The listing builds one solid part. Answer for the finished solid, in the listing's coordinates (mm). Coordinates: 2 decimals unless noted, no trailing zeros. Order: outer loops, then holes, each group sorted by start corner. A loop starts at its lowest first (then second) coordinate and runs counter-clockwise, first axis right, second up. Notation, with made-up numbers: (89, -36) -> (102, -36) arc R21 ccw to (102, -10) -> close; hole circle Ø4 at (63, 1). An arc over 180 degrees is marked (long way). Answer in a Markdown table with one row per item.
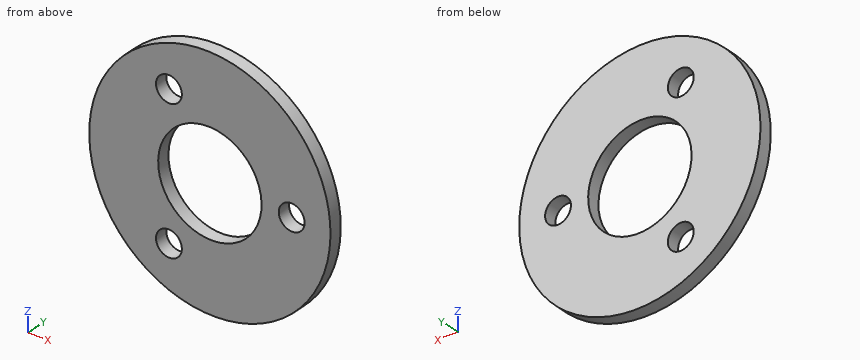
```python
from build123d import *

# Parameters (mm, degrees)
SKETCH_1_R          = 14
SKETCH_1_R_2        = 6
EXTRUDE_1_DEPTH     = 1.5
CUT_EXTRUDE_2_REACH = 21.856
SKETCH_2_R          = 1.5


with BuildPart() as part:
    # 草图1 → 凸台-拉伸1 (new body)
    with BuildSketch(Plane(origin=(0, 0, 0), x_dir=(1, 0, 0), z_dir=(0, 1, 0))):
        with Locations(Location((0, 0, 0), (0, 0, 270))):
            Circle(SKETCH_1_R)
        with Locations(Location((0, 0, 0), (0, 0, 270))):
            Circle(SKETCH_1_R_2, mode=Mode.SUBTRACT)
    extrude(amount=EXTRUDE_1_DEPTH)

    # 草图2 → 切除-拉伸2 (cut, up to next)
    with BuildSketch(Plane(origin=(0, 0, 0), x_dir=(1, 0, 0), z_dir=(0, 1, 0)), mode=Mode.PRIVATE) as cut_extrude_2_sk1:
        with Locations(Location((9.5, 0, 0), (0, 0, 270))):
            Circle(SKETCH_2_R)
    cut_extrude_2_tool1 = extrude(cut_extrude_2_sk1.sketch, amount=CUT_EXTRUDE_2_REACH, mode=Mode.PRIVATE) & part.part
    # 草图2 → 切除-拉伸2 (cut, up to next)
    with BuildSketch(Plane(origin=(0, 0, 0), x_dir=(1, 0, 0), z_dir=(0, 1, 0)), mode=Mode.PRIVATE) as cut_extrude_2_sk2:
        with Locations(Location((-4.75, -8.227241336, 0), (0, 0, 270))):
            Circle(SKETCH_2_R)
    cut_extrude_2_tool2 = extrude(cut_extrude_2_sk2.sketch, amount=CUT_EXTRUDE_2_REACH, mode=Mode.PRIVATE) & part.part
    # 草图2 → 切除-拉伸2 (cut, up to next)
    with BuildSketch(Plane(origin=(0, 0, 0), x_dir=(1, 0, 0), z_dir=(0, 1, 0)), mode=Mode.PRIVATE) as cut_extrude_2_sk3:
        with Locations(Location((-4.75, 8.227241336, 0), (0, 0, 270))):
            Circle(SKETCH_2_R)
    cut_extrude_2_tool3 = extrude(cut_extrude_2_sk3.sketch, amount=CUT_EXTRUDE_2_REACH, mode=Mode.PRIVATE) & part.part
    add(cut_extrude_2_tool1.solids().sort_by_distance((9.5, 0, 0))[0], mode=Mode.SUBTRACT)
    add(cut_extrude_2_tool2.solids().sort_by_distance((-4.75, 0, 8.227241))[0], mode=Mode.SUBTRACT)
    add(cut_extrude_2_tool3.solids().sort_by_distance((-4.75, 0, -8.227241))[0], mode=Mode.SUBTRACT)


solid = part.part
```
(1) Find the intervals of material crossed by line 1 along X through (y, z) = (1.3, 0); line 2 along Z through (x, y) = (-4.75, 0.45); line 3 along Z through (x, y) = (9.5, 0.75), in increasing order. Write a range as from..to.
Check values:
| item | result |
|---|---|
| line 1 | -14..-6, 6..8, 11..14 |
| line 2 | -13.17..-9.73, -6.73..-3.67, 3.67..6.73, 9.73..13.17 |
| line 3 | -10.28..-1.5, 1.5..10.28 |
(2) A cutting plane is placed at C-C, the plane y = 1.05. Determine the outline of the cut face in (x, z), then the cut area to 3 significant figures.
Check values:
| item | result |
|---|---|
| outline | circle Ø28 at (0, 0); hole circle Ø3 at (-4.75, -8.23); hole circle Ø3 at (-4.75, 8.23); hole circle Ø12 at (0, 0); hole circle Ø3 at (9.5, 0) |
| area | 481 mm² |
(3) A flat-ended cylindrical pin translates along its axis: pin 1 (12 mm diameter, centred on x = -3.5, z = 3, fed in from -Y). Find the tip coordinate at first contact, or state that the pin passes through.
Check values:
| item | result |
|---|---|
| pin 1 | y = 0 |
(4) A cutting plane is placed at D-D, the plane x = -4.75. Determine the outline of the cut face in (y, z).
Check values:
| item | result |
|---|---|
| outline | (0, -13.17) -> (1.5, -13.17) -> (1.5, -9.73) -> (0, -9.73) -> close; (0, -6.73) -> (1.5, -6.73) -> (1.5, -3.67) -> (0, -3.67) -> close; (0, 3.67) -> (1.5, 3.67) -> (1.5, 6.73) -> (0, 6.73) -> close; (0, 9.73) -> (1.5, 9.73) -> (1.5, 13.17) -> (0, 13.17) -> close |
(5) A cutting plane is placed at B-B, the plane z = 0. Determine the outline of the cut face in (x, y), then the cut area to 3 significant figures.
Check values:
| item | result |
|---|---|
| outline | (-14, 0) -> (-6, 0) -> (-6, 1.5) -> (-14, 1.5) -> close; (6, 0) -> (8, 0) -> (8, 1.5) -> (6, 1.5) -> close; (11, 0) -> (14, 0) -> (14, 1.5) -> (11, 1.5) -> close |
| area | 19.5 mm² |
(6) A cutting plane is placed at A-A, the plane x = 0. Determine the outline of the cut face in (y, z), then the cut area to 3 significant figures.
Check values:
| item | result |
|---|---|
| outline | (0, -14) -> (1.5, -14) -> (1.5, -6) -> (0, -6) -> close; (0, 6) -> (1.5, 6) -> (1.5, 14) -> (0, 14) -> close |
| area | 24.0 mm² |
